Can you work these out from the model? Positions are in its coordinate system, mm. A direction names the side the tool comes from. Give positions to 0.01 mm unless a question says otherwise; leave off trailing zeros. Loops run counter-clockwise (first coordinate to the right, second up) from the corner with the lowest first, then second, coordinate; pieces in that order, holes last. Notation, with made-up numbers: M -15,84 L 16,84 A12 ccw 16,104 Z; hole C -30,8.25 d6. An arc over 180 degrees is marked long. Answer as a JSON object with one key per item and string values.
Solid Edge part; units mm, degrees
sketch "Sketch1" plane through (0, 0, 0) normal (0, 0, 1) x (1, 0, 0)
  line L0 (-115.5, -115.5) -> (115.5, -115.5)
  line L1 (115.5, -115.5) -> (115.5, 87.5)
  line L2 (115.5, 87.5) -> (87.5, 115.5)
  line L3 (87.5, 115.5) -> (-87.5, 115.5)
  line L4 (-87.5, 115.5) -> (-115.5, 87.5)
  line L5 (-115.5, 87.5) -> (-115.5, -115.5)
extrude "Protrusion1" add sketch "Sketch1" along normal blind 10
sketch "Sketch2" plane through (0, 0, 10) normal (0, 0, 1) x (1, 0, 0)
  line L0 (88.7426, 118.5) -> (-88.7426, 118.5)
  line L1 (-88.7426, 118.5) -> (-118.5, 88.7426)
  line L2 (-118.5, 88.7426) -> (-118.5, -118.5)
  line L3 (-118.5, -118.5) -> (118.5, -118.5)
  line L4 (118.5, -118.5) -> (118.5, 88.7426)
  line L5 (118.5, 88.7426) -> (88.7426, 118.5)
  line L6 (87.5, 115.5) -> (-87.5, 115.5)
  line L7 (-87.5, 115.5) -> (-115.5, 87.5)
  line L8 (-115.5, 87.5) -> (-115.5, -115.5)
  line L9 (-115.5, -115.5) -> (115.5, -115.5)
  line L10 (115.5, -115.5) -> (115.5, 87.5)
  line L11 (115.5, 87.5) -> (87.5, 115.5)
extrude "Protrusion2" add sketch "Sketch2" against normal blind 41
sketch "Sketch3" plane through (-118.5, -14.8787, -10.5) normal (-1, 0, 0) x (0, -1, 0)
  line L0 (-133.3787, -20.5) -> (-14.7787, -20.5)
  line L1 (-14.7787, -20.5) -> (-14.7787, 20.5)
  line L2 (-14.7787, 20.5) -> (-133.3787, 20.5)
  line L3 (-133.3787, 20.5) -> (-133.3787, -20.5)
extrude "Cutout1" cut sketch "Sketch3" against normal blind 400
sketch "Sketch4" plane through (0, -115.5, -15.5) normal (0, 1, 0) x (-1, 0, 0)
  line L0 (-115.5, -15.5) -> (115.5, -15.5)
  line L1 (115.5, -15.5) -> (115.5, 15.5)
  line L2 (115.5, 15.5) -> (-115.5, 15.5)
  line L3 (-115.5, 15.5) -> (-115.5, -15.5)
extrude "Cutout2" cut sketch "Sketch4" against normal blind 70
1) Suppose I cut it at B-B, the plane y = -8.5. Write out the boundary of the cut face in (x, z), and give its area (3 significant figures).
Answer list:
{"outline": "M -118.5,-31 L -115.5,-31 L -115.5,0 L 115.5,0 L 115.5,-31 L 118.5,-31 L 118.5,10 L -118.5,10 Z", "area": "2,560 mm^2"}
2) For faces 5 (the flat face through (-115.5, -58, -15)), 6 (the flat face through (-2, -58, 10)), which set-ups out of +Z, -Z, +X, -X, +Y, -Y let a thin tool reach every point of the face, with its end or its side?
Answer list:
{"face 5": "-Z, +Y, -Y", "face 6": "+Z, +X, -X, +Y, -Y"}
3) Will this pin go through, and if not, where does the flat tip stop? pin 1 Ø3 at (x, y) = (82.5, -24.5) entering from -Z.
Answer list:
{"pin 1": "z = 0"}
4) Please list where these lines run through material, in increasing order: line 1 along X through (y, z) = (-29.5, -14); line 2 along Z through (x, y) = (-81, -24.5). Write a range as from..to.
Answer list:
{"line 1": "-118.5..-115.5, 115.5..118.5", "line 2": "0..10"}
5) If we mould it in two halves opening along X, with no side actions, what happens to faces 1 (the flat face through (118.5, -60, -10)), 2 (the flat face through (-2, -58, 0)), 3 (the flat face through (115.5, -60, -15)), 4 (the flat face through (-1, -118.5, 6))? For each: +X half, -X half, draft (parallel to the pull), parting line (faces both ways), or undercut.
Answer list:
{"face 1": "+X half", "face 2": "undercut", "face 3": "undercut", "face 4": "draft"}
6) Suppose I cut it at C-C, the plane x = 66. Write out the boundary of the cut face in (y, z), and give its area (3 significant figures).
Answer list:
{"outline": "M -118.5,0 L -0.1,0 L -0.1,10 L -118.5,10 Z", "area": "1,180 mm^2"}
7) Suppose I cut it at A-A, the plane z = -8. Write out the boundary of the cut face in (x, y).
Answer list:
{"outline": "M -118.5,-118.5 L -115.5,-118.5 L -115.5,-0.1 L -118.5,-0.1 Z; M 115.5,-118.5 L 118.5,-118.5 L 118.5,-0.1 L 115.5,-0.1 Z"}
